Part print with two shaded views. Sizes in mm from the minimum x, y, z corner. Round coordinates to 2 decimals unless told otherwise and drop trailing zeros. Write each loop counter-clockwise with the first axis right and the second up, starting at its lowest first coordinate (ties: lowest second). Pieces come first, ordered by that corner, then holes. Notation, with made-up numbers: (15, -2.75) -> (74, -2.75) arc R20 cw to (74, 21.25) -> close; hole circle Ø11 at (88, 41). An arc over 180 degrees is marked (long way). Return JSON: item names as keys, results as strings. Group by question number.
(1) Drill centre lines: L1, parallel to Z at x = 6.35, y = 140.25; L2, parallel to X at y = 100, z = 5.25 (1 decimal); L3, parallel to Z at x = 8.75, y = 63. Where is each one in solid material? Low to high. Write a range as from..to.
(2) Drop flat-ended pins along their axis: pin 1 Ø4 at (x, y) = (9.5, 16) entering from -Z (1 decimal); pin 2 Ø1.5 at (x, y) = (3.5, 74.5) entering from +Z; pin 3 Ø2 at (x, y) = (3, 31) entering from -Z. Give the stop position or say it passes through.
(3) Saw through at A-A (y = 78). List the corners of the cut face in (x, z).
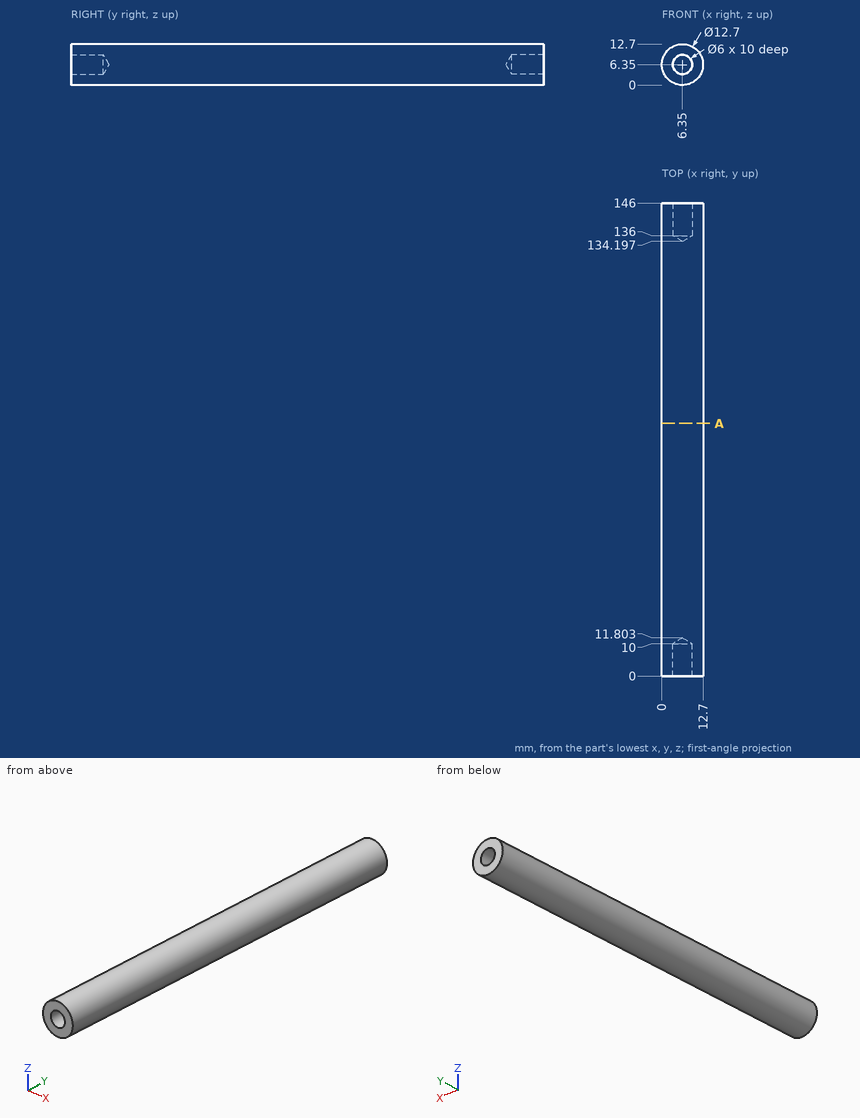
Computed values:
{
 "1": {"L1": "0..3.35, 9.35..12.7", "L2": "0.1..12.6", "L3": "0.47..12.23"},
 "2": {"pin 1": "z = 0.1", "pin 2": "z = 12.34", "pin 3": "z = 0.45"},
 "3": {"outline": "circle Ø12.7 at (6.35, 6.35)"}
}
